Check sheet for the modelled part. Datum: model origin and axes. Units: mm. A direction names the side the tool comes from. Round coordinates to 2 decimals unless told otherwise and drop trailing zeros. Write each loop counter-clockwise with the first axis right and the second up, starting at its lowest first coordinate (ties: lowest second). Pieces come first, ordered by that corner, then holes. Notation, with made-up numbers: (72.5, -34.5) -> (111.5, -34.5) arc R17 ccw to (111.5, -26.5) -> close; hole circle Ø3 at (67, 65.5). An arc over 180 degrees is marked (long way). Answer as a JSON object with one key per item and string values. Group by question number.
```python
from build123d import *

# Parameters (mm, degrees)
SKETCH1_R               = 1.65
SKETCH1_W               = 9
SKETCH1_H               = 9
SKETCH1_R_2             = 1.6
SKETCH1_R_3             = 3
SKETCH1_R_4             = 7.6
SKETCH1_R_5             = 2.6
BOSS_EXTRUDE1_DEPTH     = 3.175
FILLET1_R               = 10
CUT_EXTRUDE1_DEPTH      = 1
CUT_EXTRUDE1_DEPTH_BACK = 4.175
SKETCH3_R               = 1.65
BOSS_EXTRUDE2_DEPTH     = 3.175
FILLET2_R               = 3


with BuildPart() as part:
    # Sketch1 → Boss-Extrude1 (new body)
    with BuildSketch(Plane(origin=(0, 0, 0), x_dir=(1, 0, 0), z_dir=(0, 1, 0))):
        with BuildLine():
            Line((-51.31658538, 125.897213638), (-82.713802404, 110.430644428))
            Line((-82.713802404, 110.430644428), (-22.785408926, -11.224310227))
            ThreePointArc((-22.785408926, -11.224310227), (0, -25.4), (22.785408926, -11.224310227))
            Line((22.785408926, -11.224310227), (82.713802404, 110.430644428))
            Line((82.713802404, 110.430644428), (51.31658538, 125.897213638))
            Line((51.31658538, 125.897213638), (35.357408279, 93.5))
            Line((35.357408279, 93.5), (-35.357408279, 93.5))
            Line((-35.357408279, 93.5), (-51.31658538, 125.897213638))
        make_face()
        Polygon((-29.1997888, 81), (29.1997888, 81), (13, 48.114343343), (-13, 48.114343343), align=None, mode=Mode.SUBTRACT)
        with Locations((-8, -8)):
            Circle(SKETCH1_R, mode=Mode.SUBTRACT)
        Rectangle(SKETCH1_W, SKETCH1_H, mode=Mode.SUBTRACT)
        with Locations((-8, 8)):
            Circle(SKETCH1_R, mode=Mode.SUBTRACT)
        with Locations((-3.1, 20.76053754)):
            Circle(SKETCH1_R_2, mode=Mode.SUBTRACT)
        with Locations((8, -8)):
            Circle(SKETCH1_R, mode=Mode.SUBTRACT)
        with Locations((8, 8)):
            Circle(SKETCH1_R, mode=Mode.SUBTRACT)
        with Locations((17.5, 29.51053754)):
            Circle(SKETCH1_R_3, mode=Mode.SUBTRACT)
        with Locations((-30, 66.453060464)):
            Circle(SKETCH1_R, mode=Mode.SUBTRACT)
        with Locations((-60, 103.923048454)):
            Circle(SKETCH1_R_4, mode=Mode.SUBTRACT)
        with Locations((30, 66.453060464)):
            Circle(SKETCH1_R, mode=Mode.SUBTRACT)
        with Locations((60, 103.923048454)):
            Circle(SKETCH1_R_4, mode=Mode.SUBTRACT)
        with Locations((0, 87.25)):
            Circle(SKETCH1_R_5, mode=Mode.SUBTRACT)
        with Locations((-3.1, 38.26053754)):
            Circle(SKETCH1_R_2, mode=Mode.SUBTRACT)
    extrude(amount=BOSS_EXTRUDE1_DEPTH)

    # Fillet1
    fillet1_edges = [part.edges().sort_by_distance(p)[0] for p in [
        (51.31658538, 1.5875, -125.897213638),
        (82.713802404, 1.5875, -110.430644428),
        (-82.713802404, 1.5875, -110.430644428),
        (-51.31658538, 1.5875, -125.897213638),
    ]]
    fillet(fillet1_edges, radius=FILLET1_R)

    # Sketch2 → Cut-Extrude1 (cut, two sides)
    with BuildSketch(Plane(origin=(0, 3.175, 0), x_dir=(1, 0, 0), z_dir=(0, 1, 0))) as cut_extrude1_sk:
        Polygon((-45.79480762, 58.114343343), (-29.073580398, 58.114343343), (-12.254779912, 23.972089701), (-20.615393523, 7), align=None)
        Polygon((-63.226120316, 93.5), (-49.186747904, 65), (-40.826134293, 81.972089701), (-46.504893094, 93.5), align=None)
        Polygon((29.073580398, 58.114343343), (45.79480762, 58.114343343), (34.218483, 34.614343343), (25.857869389, 51.586433044), align=None)
        Polygon((46.504893094, 93.5), (63.226120316, 93.5), (49.186747904, 65), (40.826134293, 81.972089701), align=None)
    extrude(amount=CUT_EXTRUDE1_DEPTH, mode=Mode.SUBTRACT)
    extrude(cut_extrude1_sk.sketch, amount=-CUT_EXTRUDE1_DEPTH_BACK, mode=Mode.SUBTRACT)

    # Sketch3 → Boss-Extrude2 (add)
    with BuildSketch(Plane(origin=(0, 0, 0), x_dir=(1, 0, 0), z_dir=(0, 1, 0))):
        with BuildLine():
            Line((-69.257852251, 117.059174089), (-77.922641378, 125.361067209))
            Line((-77.922641378, 125.361067209), (-88.300007778, 114.5300808))
            Line((-88.300007778, 114.5300808), (-81.545013782, 108.057997365))
            Line((-81.545013782, 108.057997365), (-78.29478263, 101.460010992))
            ThreePointArc((-78.29478263, 101.460010992), (-78.792063776, 109.097507652), (-73.743168968, 114.849664202))
            Line((-73.743168968, 114.849664202), (-69.257852251, 117.059174089))
        make_face()
        with Locations((-78.17782959, 120.758363767)):
            Circle(SKETCH3_R, mode=Mode.SUBTRACT)
        with Locations((-83.712425003, 114.981837682)):
            Circle(SKETCH3_R, mode=Mode.SUBTRACT)
    extrude(amount=BOSS_EXTRUDE2_DEPTH)

    # Fillet2
    fillet2_edges = [part.edges().sort_by_distance(p)[0] for p in [
        (-81.545013782, 1.5875, -108.057997365),
        (-88.300007778, 1.5875, -114.5300808),
        (-77.922641378, 1.5875, -125.361067209),
        (-69.257852251, 1.5875, -117.059174089),
    ]]
    fillet(fillet2_edges, radius=FILLET2_R)


solid = part.part
```
(1) Scan lines: line 1 along Z through (x, y) = (0, 2.4); line 2 along Z through (x, y) = (42, 2.9); line 3 along Z through (x, y) = (-43, 2.9). Record each from-to range of solid material in increasing order.
(2) Access from +Z, -Z, +X, -X, +Y, -Y to the whole of each face (thin tool, end or side, straight path). Record for faces 1 (the flat face through (43.63, 1.61, -87.66)), 2 (the flat face through (-73.231, 1.565, -120.866)), 3 (the cylindrical face through (-0.396, 1.565, 25.397)).
(3) Section check A-A on z = -61. Record the cut outline in (x, y) (3 decimals).
(4) Section check B-B on y = 2.2. State how many separate pieces and enclosed holes the cut face has, then the cut area to 3 significant figures.
(5) Section check C-C on z = 13.5. Record the cut outline in (x, y) (3 decimals).
(6) Go/stop test with flat-tipped pins: pin 1 Ø3 at (x, z) = (-83.71, -114.98) entering from +Y; pin 2 Ø1.6 at (x, y) = (-38, 1.5) entering from +Z; pin 3 Ø1.6 at (x, y) = (-1, 1) entering from +Z; pin 4 Ø1.6 at (x, y) = (14, 1.5) entering from +Z. Record where each tip stops, or that it passes through.
(7) Release check for a two-part mould opening along Z. For faces 4 (the flat face through (56.305, 1.61, -79.45)), 5 (the flat face through (-5, 3.175, -34)), 6 (the flat face through (50.15, 1.57, -44.33)) record: pulls with the +Z half, pulls with the -Z half, needs draft (parallel to the pull), parting line crosses it, or undercut.
Data:
{
 "1": {"line 1": "z = -93.5 to -89.85, -84.65 to -81, -48.11 to -4.5, 4.5 to 25.4", "line 2": "z = -106.98 to -84.36, -79.59 to -58.11, -50.41 to -27.78", "line 3": "z = -109.01 to -86.39, -77.56 to -58.11, -52.44 to -29.81"},
 "2": {"face 1": "+Y, -Y", "face 2": "-Z, +Y, -Y", "face 3": "+Z, +Y, -Y"},
 "3": {"outline": "(-58.364, 0) -> (-19.348, 0) -> (-19.348, 3.175) -> (-58.364, 3.175) -> close; (19.348, 0) -> (58.364, 0) -> (58.364, 3.175) -> (19.348, 3.175) -> close"},
 "4": {"separate pieces": "1", "enclosed holes": "20", "area": "9,040 mm²"},
 "5": {"outline": "(-21.515, 0) -> (21.515, 0) -> (21.515, 3.175) -> (-21.515, 3.175) -> close"},
 "6": {"pin 1": "passes through", "pin 2": "stops at z = -18.04", "pin 3": "stops at z = 25.4", "pin 4": "stops at z = 21.7"},
 "7": {"face 4": "undercut", "face 5": "needs draft", "face 6": "pulls with the +Z half"}
}
